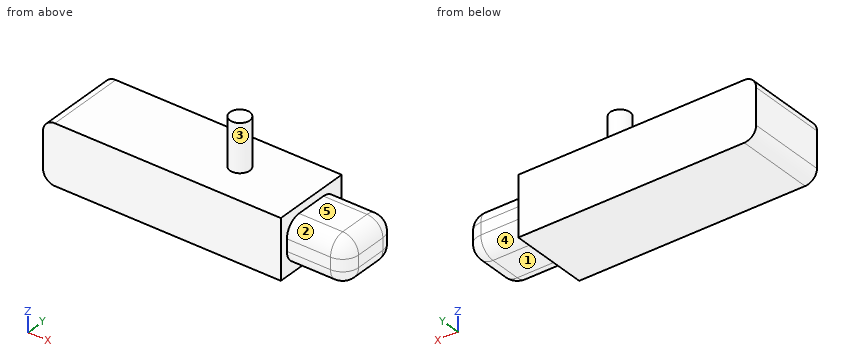
```python
from build123d import *

# Parameters (mm, degrees)
CROQUIS1_W              = 60
CROQUIS1_H              = 15
SALIENTE_EXTRUIR1_DEPTH = 20
CROQUIS2_R              = 2.5
SALIENTE_EXTRUIR2_DEPTH = 12
CROQUIS3_W              = 11
CROQUIS3_H              = 16
SALIENTE_EXTRUIR3_DEPTH = 15
REDONDEO1_R             = 4
REDONDEO2_R             = 4
REDONDEO3_R             = 3
ESCALA1_SCALE           = 2


with BuildPart() as part:
    # Croquis1 → Saliente-Extruir1 (new body)
    with BuildSketch(Plane(origin=(0, 0, 0), x_dir=(1, 0, 0), z_dir=(0, 1, 0))):
        Rectangle(CROQUIS1_W, CROQUIS1_H)
    extrude(amount=SALIENTE_EXTRUIR1_DEPTH)

    # Croquis2 → Saliente-Extruir2 (add)
    with BuildSketch(Plane.XY.offset(7.5)):
        with Locations((12, 10)):
            Circle(CROQUIS2_R)
    extrude(amount=SALIENTE_EXTRUIR2_DEPTH)

    # Croquis3 → Saliente-Extruir3 (add)
    with BuildSketch(Plane(origin=(30, 0, 0), x_dir=(0, 0, -1), z_dir=(1, 0, 0))):
        with Locations((0, 10)):
            Rectangle(CROQUIS3_W, CROQUIS3_H)
    extrude(amount=SALIENTE_EXTRUIR3_DEPTH)

    # Redondeo1
    redondeo1_edges = [part.edges().sort_by_distance(p)[0] for p in [
        (37.5, 18, 5.5),
        (37.5, 2, 5.5),
        (37.5, 2, -5.5),
        (37.5, 18, -5.5),
    ]]
    fillet(redondeo1_edges, radius=REDONDEO1_R)

    # Redondeo2
    redondeo2_edges = [part.edges().sort_by_distance(p)[0] for p in [
        (45, 18, 0),
        (45, 10, -5.5),
        (45, 10, 5.5),
        (45, 2, 0),
        (45, 16.828427125, 4.328427125),
        (45, 3.171572875, 4.328427125),
        (45, 3.171572875, -4.328427125),
        (45, 16.828427125, -4.328427125),
    ]]
    fillet(redondeo2_edges, radius=REDONDEO2_R)

    # Redondeo3
    redondeo3_edges = [part.edges().sort_by_distance(p)[0] for p in [
        (-30, 10, -7.5),
        (-30, 10, 7.5),
    ]]
    fillet(redondeo3_edges, radius=REDONDEO3_R)


with BuildPart() as part_1:
    # Escala1: scaled about (4.405278124, 10, 0.15554504)
    add(part.part.scale(ESCALA1_SCALE).moved(Location((-4.405278124, -10, -0.15554504))))


solid = part_1.part
```
For this review, take the finished solid that the model builds, in its own axes (mm). Face numbers are marked on the shaded views. A direction names the side the tool comes from. Give positions to 0.01 mm unless a question says otherwise; leave off trailing zeros. Write each loop counter-clockwise with the first axis right and the second up, starting at its lowest first coordinate (ties: lowest second). Pieces come first, ordered by that corner, then holes. Notation, with made-up numbers: M 38.25,-11 L 79.25,-11 A23 ccw 79.25,25 Z; hole C -27,-7 d7. An arc over 180 degrees is marked long. Answer as a JSON object with one key per item and string values. Group by question number.
Item 1: Consider section D-D on x = -32.5. Write out the cut boundary in (y, z).
Item 2: Consider section A-A on z = 0. Write out the cut boundary in (x, y).
Item 3: Consider section B-B on x = 66. Write out the cut boundary in (y, z).
Item 4: For pin 1 Ø6.5 at (x, z) = (61, 1) entering from -Y; pin 2 Ø12 at (y, z) = (17.5, 26.5) entering from +X; pin 3 Ø13 at (x, y) = (63.5, 9.5) entering from +Z, all flat-tipped, find the tip position at first contact; note any pin that passes through.
Item 5: Consider section C-C on y = 10. Write out the cut boundary in (x, z).
Item 6: For probe 1 along Z at (x, y) = (-26.5, -6); probe 2 along X at (y, z) = (28, -2.5); probe 3 along X at (y, z) = (9.5, 26), list the stretches that pass through material, from the lowest coordinate up. Write a range as [from, to].
Item 7: Tool access review of the marked faces 1, 2, 3, 4 and 5: name each direction out of +Z, -Z, +X, -X, +Y, -Y from which nothing blocks a thin tool from reaching the whole face with its end or side.
Check result:
{
 "1": {"outline": "M -10,-15.16 L 30,-15.16 L 30,14.84 L -10,14.84 Z"},
 "2": {"outline": "M -64.41,-10 L 55.59,-10 L 55.59,-6 L 77.59,-6 A8 ccw 85.59,2 L 85.59,18 A8 ccw 77.59,26 L 55.59,26 L 55.59,30 L -64.41,30 Z"},
 "3": {"outline": "M -6,-3.16 A8 ccw 2,-11.16 L 18,-11.16 A8 ccw 26,-3.16 L 26,2.84 A8 ccw 18,10.84 L 2,10.84 A8 ccw -6,2.84 Z"},
 "4": {"pin 1": "stops at y = -6", "pin 2": "stops at x = 24.36", "pin 3": "stops at z = 10.84"},
 "5": {"outline": "M -64.41,-9.16 A6 ccw -58.41,-15.16 L 55.59,-15.16 L 55.59,-11.16 L 77.59,-11.16 A8 ccw 85.59,-3.16 L 85.59,2.84 A8 ccw 77.59,10.84 L 55.59,10.84 L 55.59,14.84 L 24.59,14.84 L 24.59,38.84 L 14.59,38.84 L 14.59,14.84 L -58.41,14.84 A6 ccw -64.41,8.84 Z"},
 "6": {"probe 1": "z = [-15.16, 14.84]", "probe 2": "x = [-64.41, 55.59]", "probe 3": "x = [14.62, 24.57]"},
 "7": {"face 1": "-Z, +X, +Y, -Y", "face 2": "+Z, +X, -Y", "face 3": "+Z", "face 4": "-Z, +X, +Y", "face 5": "+Z, +X, +Y, -Y"}
}
